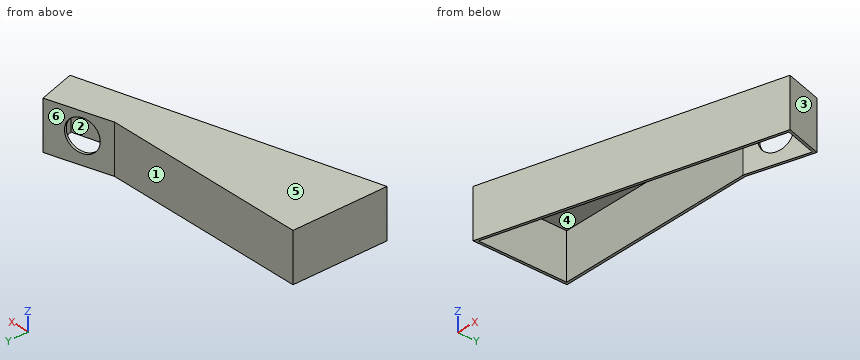
from build123d import *

# Parameters (mm, degrees)
F1_DEPTH = 38
F2_T     = -2
F3_R     = 12.5
F4_DEPTH = 25


with BuildPart() as f1:
    # F0 (on Top) → F1 (new body)
    with BuildSketch(Plane.XY):
        Polygon((160, 0), (0, 0), (0, -73.9635457095), (160, -30), (216.4829908138, -14.4800465722), (207.9198667331, 14.2718734677), align=None)
    extrude(amount=F1_DEPTH)

    # F2
    f2_openings = [f1.faces().sort_by_distance(p)[0] for p in [
        (87.670015, -24.375583, 0),
    ]]
    offset(amount=F2_T, openings=f2_openings, kind=Kind.INTERSECTION)

    # F3 (on face) → F4 (cut)
    with BuildSketch(Plane(origin=(13.0359278258, -43.7700015747, 0), x_dir=(-0.9583973347, -0.2854374694, 0), z_dir=(-0.2854374694, 0.9583973347, 0))):
        with Locations((-175.843573546, 21)):
            Circle(F3_R)
    extrude(amount=-F4_DEPTH, mode=Mode.SUBTRACT)


solid = f1.part
Input: part model. Units: mm. Frame: model coordinates. Face numbers are marked on the shaded views. A direction names the side the tool comes from. Round coordinates to 2 decimals unless told otherwise and drop trailing zeros. Order: outer loops, then holes, each group sorted by start corner. A loop starts at its lowest first (then second) coordinate and runs counter-clockwise, first axis right, second up. Notation, with made-up numbers: (1.25, -35) - (12.25, -35) arc R16 ccw to (12.25, -30) - close; hole circle Ø9 at (76.25, -38.5). An arc over 180 degrees is marked (long way). Answer as a JSON object with one key per item and string values. Group by question number.
(1) Cut plane A-A (z = 14). Return loops of the section in (x, y).
(2) Pin query (flat end, axial travel): P1, Ø1.5, axis at x = 160, z = 11, coming from the +Y side; P2, Ø19, axis at x = 98, z = 13, coming from the +Y side; P3, Ø3, axis at x = 179, z = 27, coming from the +Y side; P4, Ø8, axis at x = 178, y = -29.5, coming from the -Z side. Return the tip coordinate at first contact, or that it passes through.
(3) Draft query along X for the marked faces 4, 5 and 6. Return one class per face: released by +X, released by -X, zero draft, split by the parting line, or undercut.
(4) Cut plane B-B (x = 109.5). Return loops of the section in (y, z).
(5) Cut plane D-D (z = 25). Return loops of the section in (x, y), then the cut area to 3 significant figures.
(6) Reachability of the marked faces 1, 2 and 3 from +Z, -Z, +X, -X, +Y, -Y: full face, straight path, thin tool, end or side. Return the list, or none.
(7) Material intervals for probe 1 along Z at (x, y) = (83.5, -10.5); probe 2 along Y at (x, z) = (40.5, 17); probe 3 along Y at (x, z) = (78.5, 19.5), sorted ascending. Write a range as from..to.
(8) Cut plane C-C (y = -40.5). Return loops of the section in (x, z).
Here are the results:
{
 "1": {"outline": "(0, -73.96) - (216.48, -14.48) - (207.92, 14.27) - (191.49, 9.38) - (192.06, 7.46) - (206.57, 11.78) - (213.98, -13.09) - (2, -71.34) - (2, -2) - (160.29, -2) - (172.21, 1.55) - (171.64, 3.47) - (160, 0) - (0, 0) - close"},
 "2": {"P1": "stops at y = 0.22", "P2": "stops at y = 0", "P3": "stops at y = -22.29", "P4": "passes through"},
 "3": {"face 4": "undercut", "face 5": "zero draft", "face 6": "released by -X"},
 "4": {"outline": "(-43.88, 0) - (-41.8, 0) - (-41.8, 36) - (-2, 36) - (-2, 0) - (0, 0) - (0, 38) - (-43.88, 38) - close"},
 "5": {"outline": "(0, -73.96) - (216.48, -14.48) - (207.92, 14.27) - (192.91, 9.8) - (193.48, 7.89) - (206.57, 11.78) - (213.98, -13.09) - (2, -71.34) - (2, -2) - (160.29, -2) - (170.78, 1.13) - (170.21, 3.04) - (160, 0) - (0, 0) - close", "area": "1,010 mm^2"},
 "6": {"face 1": "+Z, -Z, -X, +Y", "face 2": "-Z", "face 3": "+Z, -Z, +X, +Y"},
 "7": {"probe 1": "z = 36..38", "probe 2": "y = -62.84..-60.76, -2..0", "probe 3": "y = -52.39..-50.32, -2..0"},
 "8": {"outline": "(0, 0) - (2, 0) - (2, 36) - (114.24, 36) - (114.24, 0) - (121.79, 0) - (121.79, 38) - (0, 38) - close"}
}
